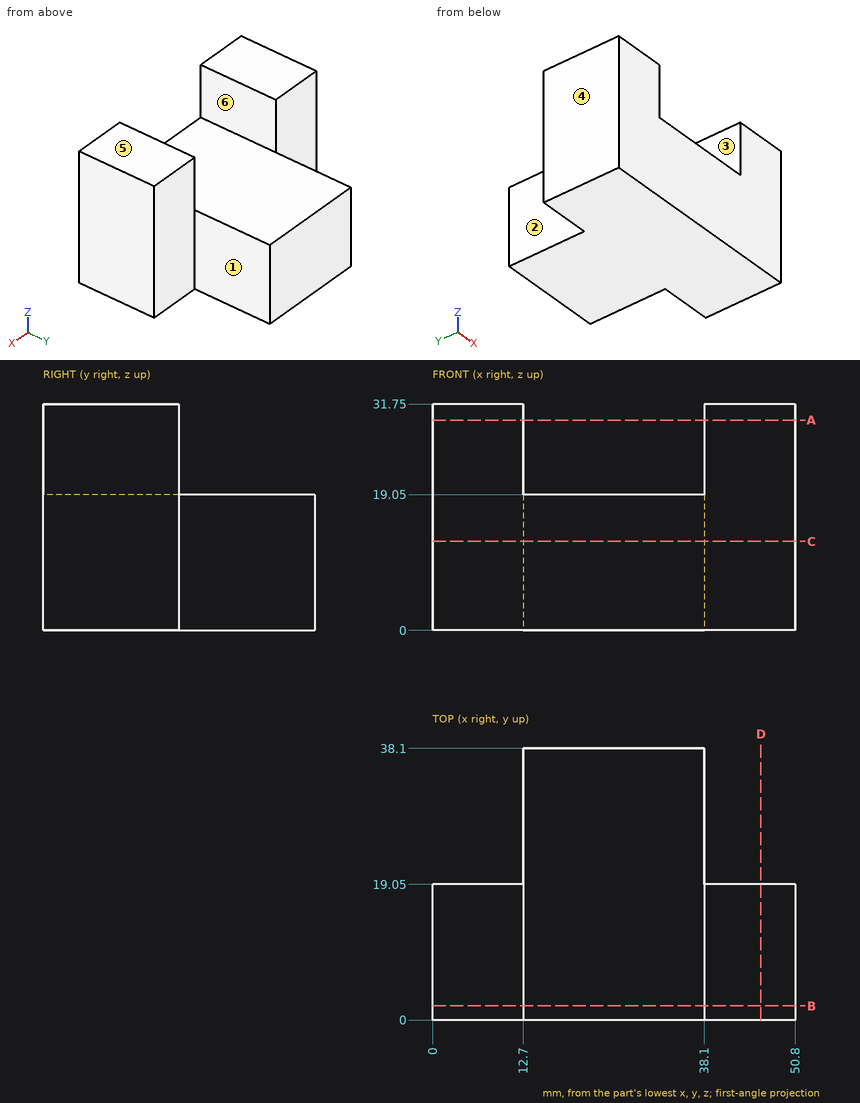
Drawing for the job (mm, zero at the part's lowest x, y, z). A direction names the side the tool comes from. Round coordinates to 2 decimals unless told otherwise and drop trailing zeros. Write each loop counter-clockwise with the first axis right and the second up, starting at its lowest first coordinate (ties: lowest second). Pieces come first, ordered by that corner, then holes.
Item 1: Mould opens along X. For the marked faces 4, 5 and 6 say: released by +X, released by -X, zero draft, split by the parting line, or undercut.
Filled in:
face 4: released by -X
face 5: zero draft
face 6: undercut
Item 2: Band-saw the part on D-D on x = 46. Write the cut outline in (y, z), then the cut area to 3 significant figures.
Filled in:
outline: (0, 0) - (19.05, 0) - (19.05, 31.75) - (0, 31.75) - close
area: 605 mm2
Item 3: Band-saw the part on A-A on z = 29.5. Write the cut outline in (x, y).
Filled in:
outline: (0, 0) - (12.7, 0) - (12.7, 19.05) - (0, 19.05) - close; (38.1, 0) - (50.8, 0) - (50.8, 19.05) - (38.1, 19.05) - close
Item 4: Drill centre lines: L1, parallel to X at y = 15, z = 22; L2, parallel to Y at x = 2, z = 24. Where is each one in solid material? Low to high.
Filled in:
L1: x = 0 to 12.7, 38.1 to 50.8
L2: y = 0 to 19.05
Item 5: Band-saw the part on B-B on y = 2. Write the cut outline in (x, z), then the cut area to 3 significant figures.
Filled in:
outline: (0, 0) - (50.8, 0) - (50.8, 31.75) - (38.1, 31.75) - (38.1, 19.05) - (12.7, 19.05) - (12.7, 31.75) - (0, 31.75) - close
area: 1,290 mm2
Item 6: Tool access for the marked faces 1, 2 and 3: list every direction of +Z, -Z, +X, -X, +Y, -Y with a clear straight run to the whole face (end or side of a thin tool).
Filled in:
face 1: +Z, -Z, +X, +Y
face 2: +Z, -Z, -X, +Y
face 3: +Z, +Y, -Y
Item 7: Drop flat-ended pins along their axis: pin 1 Ø3 at (x, z) = (24.5, 22.5) entering from +Y; pin 2 Ø4 at (x, z) = (7, 16) entering from +Y; pin 3 Ø5.5 at (y, z) = (24, 10) entering from +X; pin 4 Ø7.5 at (x, y) = (26.5, 13.5) entering from +Z. Give the stop position or say it passes through.
Filled in:
pin 1: passes through
pin 2: stops at y = 19.05
pin 3: stops at x = 38.1
pin 4: stops at z = 19.05
Item 8: Band-saw the part on C-C on z = 12.5. Write the cut outline in (x, y).
Filled in:
outline: (0, 0) - (50.8, 0) - (50.8, 19.05) - (38.1, 19.05) - (38.1, 38.1) - (12.7, 38.1) - (12.7, 19.05) - (0, 19.05) - close
